Part model, mm, in its own coordinate system. A direction names the side the tool comes from. Round coordinates to 2 decimals unless told otherwise and drop trailing zeros. Loops run counter-clockwise (first coordinate to the right, second up) from the corner with the lowest first, then second, coordinate; pieces in that order, holes last. Notation, with made-up numbers: M 66.5,53 L 105.5,53 A23 ccw 105.5,74 Z; hole C -37,60 d6. An arc over 180 degrees is marked long. Write each question's results on one line, items separated by ' | '.
from build123d import *

# Parameters (mm, degrees)
SKETCH_1_R          = 1.65
EXTRUDE_1_DEPTH     = 3
CUT_EXTRUDE_2_DEPTH = 15
SKETCH_5_R          = 2.1
CUT_EXTRUDE_4_DEPTH = 10
SKETCH_7_R          = 1.25
CUT_EXTRUDE_5_DEPTH = 10


with BuildPart() as part:
    # 草图1 → 凸台-拉伸1 (new body)
    with BuildSketch(Plane.XY):
        with BuildLine():
            Line((-22.697635701, -12.395491404), (-14.442560568, -147.364776776))
            ThreePointArc((-14.442560568, -147.364776776), (-15.823949319, -153.078271204), (-20.176817783, -157.028561017))
            ThreePointArc((-20.176817783, -157.028561017), (-47.058743214, -193.524865403), (-31.100695855, -235.950787588))
            ThreePointArc((-31.100695855, -235.950787588), (-20.888265121, -235.217514211), (-21.621538498, -225.005083476))
            ThreePointArc((-21.621538498, -225.005083476), (-32.880043508, -196.919424149), (-16.54147024, -171.451616657))
            ThreePointArc((-16.54147024, -171.451616657), (-13.7328083, -169.032706132), (-11.998184018, -165.756917888))
            ThreePointArc((-11.998184018, -165.756917888), (-0.004609984, -156.91008357), (12.004108348, -165.736350029))
            ThreePointArc((12.004108348, -165.736350029), (13.740280131, -169.004081067), (16.545879515, -171.416749859))
            ThreePointArc((16.545879515, -171.416749859), (32.911643519, -196.909572863), (21.642742476, -225.029567981))
            ThreePointArc((21.642742476, -225.029567981), (20.912749625, -235.196310232), (31.079491877, -235.926303083))
            ThreePointArc((31.079491877, -235.926303083), (47.027386385, -193.534561527), (20.172667208, -157.062392008))
            ThreePointArc((20.172667208, -157.062392008), (15.821251847, -153.112090569), (14.440433304, -147.39955722))
            Line((14.440433304, -147.39955722), (22.697635701, -12.395491404))
            ThreePointArc((22.697635701, -12.395491404), (18.150671537, -5.407168438), (10.142345541, -7.726275101))
            ThreePointArc((10.142345541, -7.726275101), (0, -12.75), (-10.142345541, -7.726275101))
            ThreePointArc((-10.142345541, -7.726275101), (-18.150671537, -5.407168438), (-22.697635701, -12.395491404))
        make_face()
        with Locations((-11.313708499, -11.313708499)):
            Circle(SKETCH_1_R, mode=Mode.SUBTRACT)
        with Locations((0, -16)):
            Circle(SKETCH_1_R, mode=Mode.SUBTRACT)
        with Locations((11.313708499, -11.313708499)):
            Circle(SKETCH_1_R, mode=Mode.SUBTRACT)
    extrude(amount=EXTRUDE_1_DEPTH)

    # 草图4 → 切除-拉伸2 (cut)
    with BuildSketch(Plane(origin=(0, 0, 0), x_dir=(-1, 0, 0), z_dir=(0, 0, -1))):
        with BuildLine():
            Line((-13.715926625, -28.201870805), (-10.113702702, -87.097711346))
            ThreePointArc((-10.113702702, -87.097711346), (-9.904103863, -88.030297779), (-9.411801117, -88.849618921))
            Line((-9.411801117, -88.849618921), (-2.292502811, -97.284018261))
            ThreePointArc((-2.292502811, -97.284018261), (0, -98.348965067), (2.292502811, -97.284018261))
            Line((2.292502811, -97.284018261), (9.411801117, -88.849618921))
            ThreePointArc((9.411801117, -88.849618921), (9.904103863, -88.030297779), (10.113702702, -87.097711346))
            Line((10.113702702, -87.097711346), (13.715926625, -28.201870805))
            ThreePointArc((13.715926625, -28.201870805), (12.496725506, -25.600326268), (9.649370007, -25.216852668))
            ThreePointArc((9.649370007, -25.216852668), (0, -27), (-9.649370007, -25.216852668))
            ThreePointArc((-9.649370007, -25.216852668), (-12.496725506, -25.600326268), (-13.715926625, -28.201870805))
        make_face()
    extrude(amount=-CUT_EXTRUDE_2_DEPTH, mode=Mode.SUBTRACT)

    # 草图5 → 切除-拉伸4 (cut)
    with BuildSketch(Plane.XY.offset(3)):
        with Locations((0, -188.402692504)):
            Circle(SKETCH_5_R)
        with Locations((0, -118.402692504)):
            Circle(SKETCH_5_R)
    extrude(amount=-CUT_EXTRUDE_4_DEPTH, mode=Mode.SUBTRACT)

    # 草图7 → 切除-拉伸5 (cut)
    with BuildSketch(Plane.XY.offset(3)):
        with Locations((0, -163.538416724)):
            Circle(SKETCH_7_R)
        with Locations((23.461747754, -172.07779455)):
            Circle(SKETCH_7_R)
        with Locations((35.945482985, -193.700258239)):
            Circle(SKETCH_7_R)
        with Locations((31.609927238, -218.288416724)):
            Circle(SKETCH_7_R)
        with Locations((12.483735231, -234.337197383)):
            Circle(SKETCH_7_R)
        with Locations((-12.483735231, -234.337197383)):
            Circle(SKETCH_7_R)
        with Locations((-31.609927238, -218.288416724)):
            Circle(SKETCH_7_R)
        with Locations((-35.945482985, -193.700258239)):
            Circle(SKETCH_7_R)
        with Locations((-23.461747754, -172.07779455)):
            Circle(SKETCH_7_R)
    extrude(amount=-CUT_EXTRUDE_5_DEPTH, mode=Mode.SUBTRACT)


solid = part.part
Item 1: Band-saw the part on C-C on y = -106.5. Give the cut face in (x, z), and give its area (3 significant figures).
Filled sheet:
outline: M -16.94,0 L 16.94,0 L 16.94,3 L -16.94,3 Z | area: 102 mm^2
Item 2: Drop flat-ended pins along their axis: P1, Ø4, axis at x = -11.31, y = -11.31, coming from the -Z side; P2, Ø1, axis at x = 24, z = 1.5, coming from the -Y side; P3, Ø1.5, axis at y = -175.5, z = 1, coming from the +X side. Give the stop position or say it passes through.
Filled sheet:
P1: z = 0 | P2: y = -237.44 | P3: x = 41.09
Item 3: Wall check: L1, parallel to Y at x = 0, z = 2.3; L2, parallel to Y at x = 7, z = 1.1; L3, parallel to X at y = -17, z = 0.85. Give the ranges that are in metal, low to high.
Filled sheet:
L1: -156.91 to -120.5, -116.3 to -98.35, -27 to -17.65, -14.35 to -12.75 | L2: -159.04 to -91.71, -26.08 to -10.66 | L3: -22.42 to -1.31, 1.31 to 22.42
Item 4: Band-saw the part on B-B on z = 2.05. Count the separate pieces of the cut face and the enclosed holes in it, and give its area (3 significant figures).
Filled sheet:
separate pieces: 1 | enclosed holes: 11 | area: 6,490 mm^2
Item 5: Two-plate mould, pull along Y, no slides. Class faces 5 (the cylindrical face through (20.81, -235.075, 1.479)), 6 (the flat face through (0, -129, 3)), 7 (the cylindrical face through (-0.228, -156.912, 1.479)): +Y half, -Y half, draft (parallel to the pull), parting line (faces both ways), or undercut.
Filled sheet:
face 5: undercut | face 6: draft | face 7: -Y half
Item 6: Which spindle directions (+Z, -Z, +X, -X, +Y, -Y) get a long thin tool onto all of the face, cutting with end or side? Do faces 1 (the flat face through (5.9, -93.01, 1.48)), 2 (the cylindrical face through (-13.765, -169.073, 1.479)), 3 (the flat face through (-18.628, -78.935, 1.479)), 4 (the flat face through (18.51, -80.84, 1.48)). Say none if no direction does.
Filled sheet:
face 1: +Z, -Z | face 2: +Z, -Z, -Y | face 3: +Z, -Z, -X | face 4: +Z, -Z, +X
Item 7: Band-saw the part on D-D on y = -150. Give the cut face in (x, z).
Filled sheet:
outline: M -14.63,0 L 14.62,0 L 14.62,3 L -14.63,3 Z
Item 8: Band-saw the part on A-A on x = 6. Give the cut face in (y, z).
Filled sheet:
outline: M -158.43,0 L -92.89,0 L -92.89,3 L -158.43,3 Z; M -26.32,0 L -11.25,0 L -11.25,3 L -26.32,3 Z
